from build123d import *

# Parameters (mm, degrees)
F0_R     = 57.15
F0_R_2   = 5
F1_DEPTH = 15
F2_R     = 9.345245
F2_R_2   = 5.107746
F3_DEPTH = 30
F4_R     = 1.5
F5_DEPTH = 12.7
F6_R     = 2.25
F7_DEPTH = 10


with BuildPart() as f1:
    # F0 (on Front) → F1 (new body)
    with BuildSketch(Plane.XZ):
        Circle(F0_R)
        Circle(F0_R_2, mode=Mode.SUBTRACT)
    extrude(amount=F1_DEPTH)

    # F2 (on face) → F3 (join)
    with BuildSketch(Plane.XZ.offset(15)):
        Circle(F2_R)
        Circle(F2_R_2, mode=Mode.SUBTRACT)
    extrude(amount=F3_DEPTH)

    # F4 (on Top) → F5 (cut, symmetric)
    with BuildSketch(Plane.XY):
        with Locations((0, -21.58)):
            Circle(F4_R)
    extrude(amount=F5_DEPTH, both=True, mode=Mode.SUBTRACT)

    # F6 (on face) → F7 (cut)
    with BuildSketch(Plane(origin=(0, 0, 0), x_dir=(-1, 0, 0), z_dir=(0, 1, 0))):
        with Locations((0, 10)):
            Circle(F6_R)
        with Locations((7.071068, 7.071068)):
            Circle(F6_R)
        with Locations((10, 0)):
            Circle(F6_R)
        with Locations((0, -10)):
            Circle(F6_R)
        with Locations((7.071068, -7.071068)):
            Circle(F6_R)
        with Locations((-7.071068, -7.071068)):
            Circle(F6_R)
        with Locations((-10, 0)):
            Circle(F6_R)
        with Locations((-7.071068, 7.071068)):
            Circle(F6_R)
    extrude(amount=-F7_DEPTH, mode=Mode.SUBTRACT)


solid = f1.part
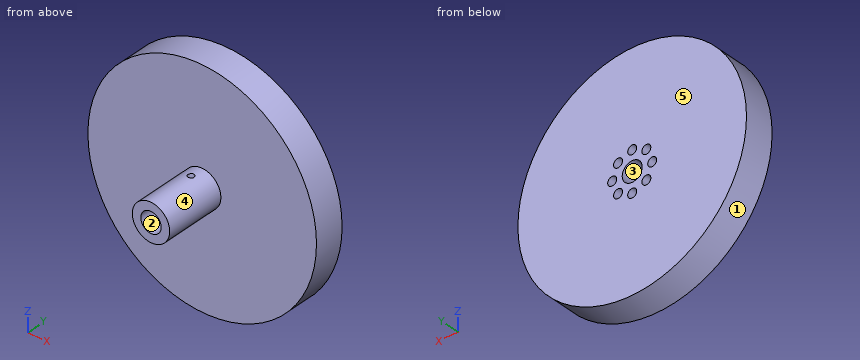
The listing builds one solid part. Answer for the finished solid, in the listing's coordinates (mm). Face numbers are marked on the shaded views. A direction names the side the tool comes from. Give positions to 0.01 mm unless a question says otherwise; leave off trailing zeros. Order: outer loops, then holes, each group sorted by start corner. A loop starts at its lowest first (then second) coordinate and runs counter-clockwise, first axis right, second up. Notation, with made-up numbers: (-28.75, 55) - (10.25, 55) arc R9 cw to (10.25, 59) - close; hole circle Ø1 at (62.5, 87). An arc over 180 degrees is marked (long way). Use one line per item in the form item = value.
1) The mould has two halves that part along Z. Classify the marked faces 3, 4 and 5: released by +Z, released by -Z, zero draft, split by the parting line, or undercut.
Verdict:
face_3 = undercut
face_4 = split by the parting line
face_5 = zero draft
2) Consider probe 1 along Z at (x, y) = (0, -4.5); probe 2 along Z at (x, y) = (0, -36.5); probe 3 along Z at (x, y) = (-11, -3.5). Determine where each line is inside the solid, lowest interval first. Write a range as [from, to].
Verdict:
probe_1 = [-57.15, -12.25], [-7.75, -5], [5, 7.75], [12.25, 57.15]
probe_2 = [-9.35, -5.11], [5.11, 9.35]
probe_3 = [-56.08, -2.02], [2.02, 56.08]
3) Find section B-B on x = 0. Give the number of separate pieces and of enclosed holes in the cut face, and give its area (3 significant figures).
Verdict:
separate_pieces = 4
enclosed_holes = 0
area = 1,700 mm^2
4) Each of these flat-tipped pins is pushed along its axis until it touches: pin 1 (5 mm diameter, centred on y = -6.5, z = 12, fed in from -X); pin 2 (8 mm diameter, centred on y = -18, z = -35, fed in from +X); pin 3 (8 mm diameter, centred on y = -17, z = -21, fed in from -X). Where does it stop, or does it pass through?
Verdict:
pin_1 = -56.35
pin_2 = 47.11
pin_3 = -54.39
5) Find section A-A on z = 0. Determine the outline of the cut face in (x, y).
Verdict:
outline = (-57.15, -15) - (-9.35, -15) - (-9.35, -45) - (-5.11, -45) - (-5.11, -15) - (-5, -15) - (-5, 0) - (-7.75, 0) - (-7.75, -10) - (-12.25, -10) - (-12.25, 0) - (-57.15, 0) - close; (5, -15) - (5.11, -15) - (5.11, -45) - (9.35, -45) - (9.35, -15) - (57.15, -15) - (57.15, 0) - (12.25, 0) - (12.25, -10) - (7.75, -10) - (7.75, 0) - (5, 0) - close
6) For the marked faces 1 and 2, determine the directions among +Z, -Z, +X, -X, +Y, -Y from which every point of the face is accessible in a straight line to the end or side of a thin tool.
Verdict:
face_1 = +Y, -Y
face_2 = -Y
7) Find section D-D on y = -21.58. Determine the outline of the cut face in (x, z).
Verdict:
outline = (-1.5, -9.22) - (-1.5, -4.88) arc R5.11 cw to (-1.5, 4.88) - (-1.5, 9.22) arc R9.35 ccw to start; (1.5, -9.22) arc R9.35 ccw to (1.5, 9.22) - (1.5, 4.88) arc R5.11 cw to (1.5, -4.88) - close
